from build123d import *

# Parameters (mm, degrees)
F0_R      = 12
F0_R_2    = 33.5
F1_DEPTH  = 50
F4_DEPTH  = 25
F5_W      = 12
F5_H      = 25
F6_DEPTH  = 1
F7_DEPTH  = 12
F8_R      = 3.429
F9_DEPTH  = 30
F10_R     = 1.75
F11_DEPTH = 25
F12_W     = 6
F12_H     = 8.7619052733
F13_DEPTH = 55
F15_DEPTH = 52
F17_DEPTH = 50
F18_W     = 81.3058614731
F18_H     = 161.7973074317
F19_DEPTH = 50
F20_W     = 42.0657843351
F20_H     = 29.0236644447
F21_DEPTH = 250


with BuildPart() as f1:
    # F0 (on Top) → F1 (new body)
    with BuildSketch(Plane.XY):
        with BuildLine():
            ThreePointArc((34.510392045, 31.4329896907), (0, 87), (-34.510392045, 31.4329896907))
            Line((-34.510392045, 31.4329896907), (-15.238354929, -7.5360824742))
            ThreePointArc((-15.238354929, -7.5360824742), (0, -17), (15.238354929, -7.5360824742))
            Line((15.238354929, -7.5360824742), (34.510392045, 31.4329896907))
        make_face()
        Circle(F0_R, mode=Mode.SUBTRACT)
        with Locations((0, 48.5)):
            Circle(F0_R_2, mode=Mode.SUBTRACT)
    extrude(amount=F1_DEPTH)

    # F3 (on offset) → F4 (cut)
    with BuildSketch(Plane.XZ.offset(-87)):
        with BuildLine():
            add(Edge.make_bspline(
                [(17.5, 50), (17.5, 73), (0, 73), (-17.5, 73), (-17.5, 50)],
                knots=[1.5707963268, 1.5707963268, 1.5707963268, 3.1415926536, 3.1415926536, 4.7123889804, 4.7123889804, 4.7123889804], degree=2, weights=[1, 0.7071067812, 1, 0.7071067812, 1]))
            Line((-17.5, 50), (17.5, 50))
        make_face()
        with BuildLine():
            Line((17.5, 50), (-17.5, 50))
            add(Edge.make_bspline(
                [(-17.5, 50), (-17.5, 27), (0, 27)],
                knots=[4.7123889804, 4.7123889804, 4.7123889804, 6.2831853072, 6.2831853072, 6.2831853072], degree=2, weights=[1, 0.7071067812, 1]))
            add(Edge.make_bspline(
                [(0, 27), (17.5, 27), (17.5, 50)],
                knots=[0, 0, 0, 1.5707963268, 1.5707963268, 1.5707963268], degree=2, weights=[1, 0.7071067812, 1]))
        make_face()
    extrude(amount=F4_DEPTH, mode=Mode.SUBTRACT)

    # F5 (on offset) → F6 (join)
    with BuildSketch(Plane.XZ.offset(-87)):
        with Locations((0, 12.5)):
            Rectangle(F5_W, F5_H)
    extrude(amount=F6_DEPTH)

    # F5 (on offset) → F7 (join)
    with BuildSketch(Plane.XZ.offset(-87)):
        with Locations((0, 12.5)):
            Rectangle(F5_W, F5_H)
    extrude(amount=-F7_DEPTH)

    # F8 (on Right) → F9 (cut, symmetric)
    with BuildSketch(Plane.YZ):
        with Locations((0, 12.5)):
            Circle(F8_R)
    extrude(amount=F9_DEPTH, both=True, mode=Mode.SUBTRACT)

    # F10 (on face) → F11 (cut)
    with BuildSketch(Plane(origin=(-6, 0, 0), x_dir=(0, -1, 0), z_dir=(-1, 0, 0))):
        with Locations((-92.7647968698, 12.5)):
            Circle(F10_R)
    extrude(amount=-F11_DEPTH, mode=Mode.SUBTRACT)

    # F12 (on face) → F13 (cut)
    with BuildSketch(Plane.XY.offset(50)):
        with Locations((0, 13.4115335532)):
            Rectangle(F12_W, F12_H)
    extrude(amount=-F13_DEPTH, mode=Mode.SUBTRACT)

    # F14 (on face) → F15 (cut)
    with BuildSketch(Plane.XY.offset(50)):
        with BuildLine():
            ThreePointArc((10.7564858322, -5.3195876289), (0, -12), (-10.7564858322, -5.3195876289))
            Line((-10.7564858322, -5.3195876289), (-15.238354929, -7.5360824742))
            ThreePointArc((-15.238354929, -7.5360824742), (0, -17), (15.238354929, -7.5360824742))
            Line((15.238354929, -7.5360824742), (10.7564858322, -5.3195876289))
        make_face()
    extrude(amount=-F15_DEPTH, mode=Mode.SUBTRACT)

    # F16 (on Top) → F17 (join)
    with BuildSketch(Plane.XY):
        Polygon((-10.7564858322, -5.3195876289), (-15.238354929, -7.5360824742), (-13.0218600836, -12.017951571), (-8.5399909869, -9.8014567256), align=None)
        Polygon((13.0218600836, -12.017951571), (15.238354929, -7.5360824742), (10.7564858322, -5.3195876289), (8.5399909869, -9.8014567256), align=None)
    extrude(amount=F17_DEPTH)

    # F18 (on Top) → F19 (cut)
    with BuildSketch(Plane.XY):
        with Locations((40.6529307365, 33.7636955082)):
            Rectangle(F18_W, F18_H)
    extrude(amount=F19_DEPTH, mode=Mode.SUBTRACT)

    # F20 (on Front) → F21 (cut, symmetric)
    with BuildSketch(Plane.XZ):
        with Locations((-21.0328921676, 39.5118322223)):
            Rectangle(F20_W, F20_H)
    extrude(amount=F21_DEPTH, both=True, mode=Mode.SUBTRACT)


solid = f1.part
Here's how the part is built. I have some questions about the finished solid (model axes, mm). A direction names the side the tool comes from. Give positions to 0.01 mm unless a question says otherwise; leave off trailing zeros. Write each loop counter-clockwise with the first axis right and the second up, starting at its lowest first coordinate (ties: lowest second). Pieces come first, ordered by that corner, then holes. Notation, with made-up numbers: (-30, 57) -> (12, 57) arc R16 ccw to (12, 65) -> close; hole circle Ø8 at (80.25, 51.5). An arc over 180 degrees is marked (long way). Use one line per item in the form item = value. Start each with the question number.
1. Thinking about a two-plate mould opening in Z: for faces 1 (the face through (0, 90, 12)), 2 (the face through (-26, 27, 0)), 3 (the face through (-3.042, 91.096, 13.026)), which applies, +Z half, -Z half, draft (parallel to the pull), parting line (faces both ways), or undercut?
2. Imagine slicing it at C-C on y = -1. List the corners of the cut face in (x, z) for me.
3. Will these pins go through, and if not, where does the flat tip stop? pin 1 Ø2 at (x, z) = (-12.5, 7) entering from +Y; pin 2 Ø10 at (y, z) = (93, 18.5) entering from -X; pin 3 Ø12 at (y, z) = (64, 6.5) entering from -X; pin 4 Ø12 at (x, y) = (-25.5, 42) entering from -Z.
4. Imagine slicing it at B-B on x = -19. List the corners of the cut face in (y, z) for me, plus the area to 3 significant figures.
5. Imagine slicing it at A-A on z = 2.25. List the corners of the cut face in (x, y) for me.
6. On a 3-axis mill with a long thin cutter (end or side, diameter ignored), from which of +Z, -Z, +X, -X, +Y, -Y can I reach the whole of each face in a straight line? I mean faces 4 (the face through (-3, 13, 13)), 5 (the face through (-9.633, -7.592, 12.325)), 6 (the face through (-33.96, 66.64, 12.32)), 7 (the face through (-6, 95, 12)). Say none if no direction works.
7. If I drill on L1, parallel to Y at x = -14, z = 12.5; L2, parallel to Z at x = -14.75, y = 0; L3, parallel to Y at x = -31, z = 5, over which ranges is the centre line in solid material (lowest first)?
8. Imagine slicing it at D-D on x = -14. List the corners of the cut face in (y, z) for me.
Entries:
q1.face_1 = draft
q1.face_2 = -Z half
q1.face_3 = undercut
q2.outline = (-18.47, 0) -> (-11.96, 0) -> (-11.96, 9.22) -> (-18.47, 9.22) -> close; (-18.47, 15.78) -> (-11.96, 15.78) -> (-11.96, 25) -> (-18.47, 25) -> close
q3.pin_1 = 85.24
q3.pin_2 = -6
q3.pin_3 = -37.31
q3.pin_4 = through
q4.outline = (0.07, 0) -> (20.91, 0) -> (20.91, 25) -> (0.07, 25) -> (0.07, 15.93) arc R3.43 cw to (0.07, 9.07) -> close; (76.09, 0) -> (81.99, 0) -> (81.99, 25) -> (76.09, 25) -> close
q4.area = 650 mm²
q5.outline = (-34.51, 31.43) -> (-13.02, -12.02) -> (-8.54, -9.8) -> (-10.76, -5.32) arc R12 cw to (-3, 11.62) -> (-3, 15.13) arc R33.5 cw to (0, 82) -> (0, 99) -> (-6, 99) -> (-6, 86.53) arc R38.5 ccw to start
q6.face_4 = +Z, -Z, +X, -Y
q6.face_5 = +Z, -Z, +X
q6.face_6 = +Z, -Z, -X
q6.face_7 = +Z, -Z, -X, +Y
q7.L1 = -10.04 to -3.43, 3.43 to 18.07, 78.93 to 84.36
q7.L2 = 0 to 9.07, 15.93 to 25
q7.L3 = 24.33 to 35.8, 61.2 to 71.33
q8.outline = (-10.04, 0) -> (18.07, 0) -> (18.07, 25) -> (-10.04, 25) -> close; (78.93, 0) -> (84.36, 0) -> (84.36, 25) -> (78.93, 25) -> close; hole circle Ø6.86 at (0, 12.5)
